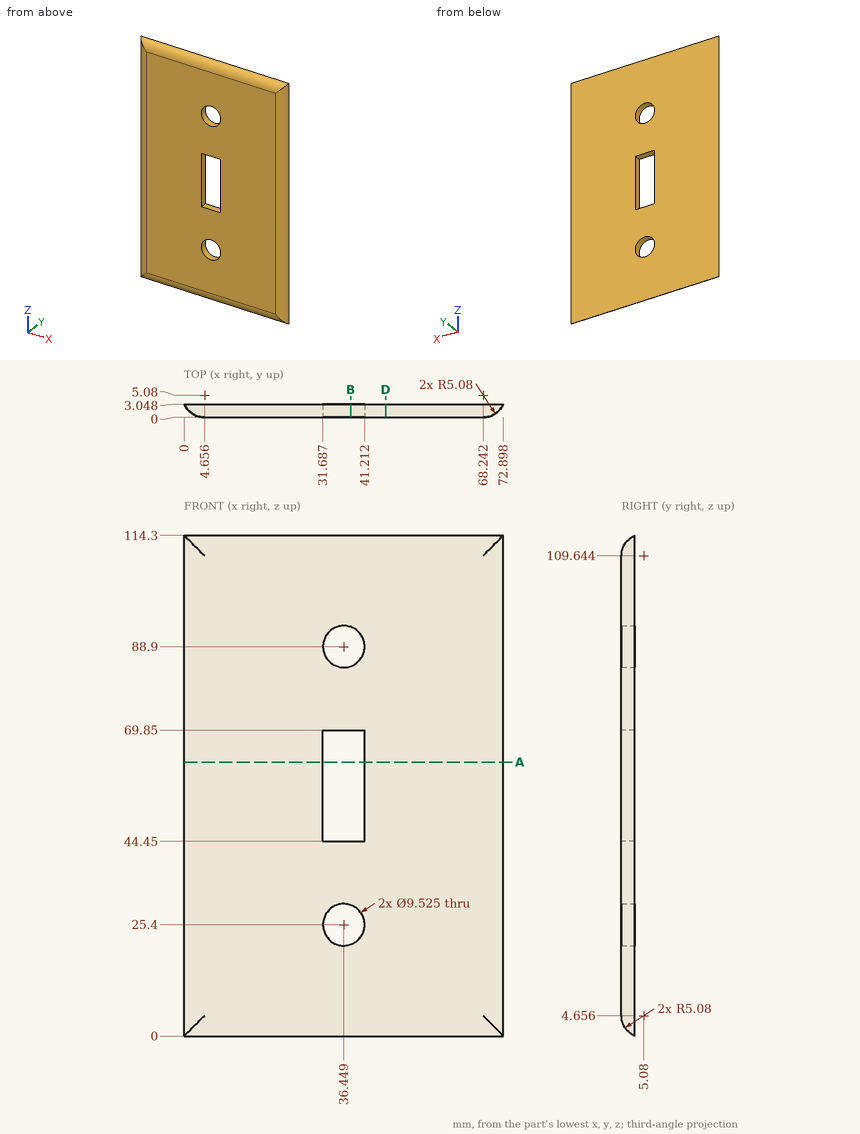
The figure shows three views and two pictorial views of one solid part (mm, origin at its lowest corner). Answer the questions. Coordinates: 2 decimals unless noted, no trailing zeros. Write each loop counter-clockwise with the first axis right and the second up, starting at its lowest first coordinate (ties: lowest second). Pieces come first, ordered by that corner, then holes. Notation, with made-up numbers: (70, -23) -> (106, -23) arc R9 ccw to (106, -16) -> close; hole circle Ø8 at (51.5, 35.25). An arc over 180 degrees is marked (long way). Return JSON: item names as keys, results as strings.
1. A cutting plane is placed at D-D (x = 46). Determine the outline of the cut face in (y, z) (1 decimal).
Found:
{"outline": "(0, 4.7) arc R5.1 ccw to (3, 0) -> (3, 114.3) arc R5.1 ccw to (0, 109.6) -> close"}
2. A cutting plane is placed at A-A (z = 62.5). Determine the outline of the cut face in (x, y) (1 decimal), and give its area (3 significant figures).
Found:
{"outline": "(0, 3) arc R5.1 ccw to (4.7, 0) -> (31.7, 0) -> (31.7, 3) -> close; (41.2, 0) -> (68.2, 0) arc R5.1 ccw to (72.9, 3) -> (41.2, 3) -> close", "area": "185 mm2"}
3. Find the intervals of material crossed by line 1 along X through (y, z) = (1.9, 46) (1 decimal); line 2 along X through (y, z) = (0.95, 88.9) (1 decimal); line 3 along X through (y, z) = (0.4, 77) (1 decimal), in increasing order. Write a range as from..to.
Found:
{"line 1": "0.7..31.7, 41.2..72.2", "line 2": "1.7..31.7, 41.2..71.2", "line 3": "2.7..70.2"}
4. Each of these flat-tipped pins is pushed along its axis until it touches: P1, Ø1, axis at x = 26, y = 2, coming from the -Z side; P2, Ø0.9, axis at y = 1.5, z = 61, coming from the +X side; P3, Ø1, axis at y = 1, z = 43.5, coming from the +X side (1 decimal). Where does it stop, or does it pass through?
Found:
{"P1": "z = 0.28", "P2": "x = 72.24", "P3": "x = 71.8"}
5. A cutting plane is placed at B-B (x = 38). Give the number of separate pieces and of enclosed holes in the cut face, and give its area (3 significant figures).
Found:
{"separate pieces": "4", "enclosed holes": "0", "area": "208 mm2"}
